Here's how the part is built. I have some questions about the finished solid (model axes, mm). Round coordinates to 2 decimals unless told otherwise and drop trailing zeros. Order: outer loops, then holes, each group sorted by start corner. A loop starts at its lowest first (then second) coordinate and runs counter-clockwise, first axis right, second up. Notation, with made-up numbers: M 32,28.25 L 46,28.25 A23 ccw 46,57.25 Z; hole C -32.5,4 d5. An arc over 180 degrees is marked long. Use one line per item in the form item = value. Start each with the question number.
```python
from build123d import *

# Parameters (mm, degrees)
CUT_EXTRUDE1_DEPTH  = 0.32
CIRPATTERN1_COUNT   = 4
DRAFT2_ANGLE        = 5
SKETCH8_R           = 0.8
BOSS_EXTRUDE1_DEPTH = 0.26
BOSS_EXTRUDE1_DRAFT = -45


with BuildPart() as part:
    # Sketch3 → Revolve1 (revolve)
    with BuildSketch(Plane(origin=(0, 0, 0), x_dir=(0, 0, -1), z_dir=(1, 0, 0)), mode=Mode.PRIVATE) as revolve1_sk:
        Polygon((-0.96, 0), (-0.96, 1.5), (-0.26, 0.8), (-0.26, 0), align=None)
    revolve(revolve1_sk.sketch.rotate(Axis((0, 0, 0.96), (0, 0, -1)), 180), axis=Axis((0, 0, 0.96), (0, 0, -1)))

    # Sketch5 → Revolve2 (revolve)
    with BuildSketch(Plane(origin=(0, 0, 0), x_dir=(0, 0, -1), z_dir=(1, 0, 0))):
        Polygon((17.04, 0), (-0.26, 0), (-0.26, 0.8), (16.7635, 0.8), (17.04, 0.5235), align=None)
    revolve(axis=Axis((0, 0, -17.04), (0, 0, 1)))

    # Sketch4 → Cut-Extrude1 (cut)
    with BuildSketch(Plane.XY.offset(0.96)):
        with BuildLine():
            Line((0, 0), (0.9271, 0))
            ThreePointArc((0.9271, 0), (0.92214099, 0.095762227), (0.907317012, 0.1905))
            Line((0.907317012, 0.1905), (0.548908506, 0.1905))
            Line((0.548908506, 0.1905), (0.295475421, 0.295475421))
            Line((0.295475421, 0.295475421), (0.1905, 0.548908506))
            Line((0.1905, 0.548908506), (0.1905, 0.907317012))
            ThreePointArc((0.1905, 0.907317012), (0.095762227, 0.92214099), (0, 0.9271))
            Line((0, 0.9271), (0, 0))
        make_face()
    cut_extrude1 = extrude(amount=-CUT_EXTRUDE1_DEPTH, mode=Mode.SUBTRACT)

    # CirPattern1: Cut-Extrude1 ×4 about axis
    cirpattern1_axis = Axis((0, 0, 0), (0, 0, 1))
    for i in range(1, CIRPATTERN1_COUNT):
        add(cut_extrude1.rotate(cirpattern1_axis, i * 360 / CIRPATTERN1_COUNT), mode=Mode.SUBTRACT)

    # Draft2
    draft2_faces = [part.faces().sort_by_distance(p)[0] for p in [
        (-0.728112759, 0.1905, 0.8),
        (-0.422191963, 0.24298771, 0.8),
        (-0.24298771, 0.422191963, 0.8),
        (-0.1905, 0.728112759, 0.8),
        (0.1905, 0.728112759, 0.8),
        (0.24298771, 0.422191963, 0.8),
        (0.422191963, 0.24298771, 0.8),
        (0.728112759, 0.1905, 0.8),
        (0.728112759, -0.1905, 0.8),
        (0.422191963, -0.24298771, 0.8),
        (0.24298771, -0.422191963, 0.8),
        (0.1905, -0.728112759, 0.8),
        (-0.1905, -0.728112759, 0.8),
        (-0.24298771, -0.422191963, 0.8),
        (-0.422191963, -0.24298771, 0.8),
        (-0.728112759, -0.1905, 0.8),
    ]]
    draft(draft2_faces, Plane(origin=(0, 0, 0.96), x_dir=(0, 1, 0), z_dir=(0, 0, 1)), DRAFT2_ANGLE)


with BuildPart() as body_2:
    # Split1: the piece on the far side of the plane
    add(part.part)
    split(bisect_by=Plane(origin=(0, 0, 0.26), x_dir=(0, -1, 0), z_dir=(0, 0, -1)), keep=Keep.BOTTOM)


with BuildPart() as part_1:
    add(part.part)

    # Split1
    split(bisect_by=Plane(origin=(0, 0, 0.26), x_dir=(0, -1, 0), z_dir=(0, 0, -1)), keep=Keep.TOP)


with BuildPart() as body_2_1:
    add(body_2.part)

    # Combine1: union part
    add(part_1.part)


with BuildPart() as boss_extrude1_tool:
    # Sketch8 → Boss-Extrude1 (with draft: the straight prism first)
    with BuildSketch(Plane.XY.offset(0.26)):
        with Locations(Location((0, 0, 0), (0, 0, 90))):
            Circle(SKETCH8_R)
    extrude(amount=-BOSS_EXTRUDE1_DEPTH)
    # Boss-Extrude1: the draft: its side faces are tilted about the plane it starts from
    boss_extrude1_sides = [boss_extrude1_tool.faces().sort_by_distance(p)[0] for p in [
        (0, -0.8, 0.13),
    ]]
    draft(boss_extrude1_sides, Plane.XY.offset(0.26), BOSS_EXTRUDE1_DRAFT)


with BuildPart() as body_2_2:
    add(body_2_1.part)

    # Boss-Extrude1: add boss_extrude1_tool
    add(boss_extrude1_tool.part)


solid = body_2_2.part
```
1) Will this pin go through, and if not, where does the flat tip stop? pin 1 Ø1 at (x, z) = (-1, -14) entering from -Y.
2) If we mould it in two halves opening along Y, with no side actions, what happens to faces 1 (the cylindrical face through (0.49, -0.63, -8.37)), 2 (the flat face through (0, 0, -17.04)), 3 (the flat face through (0, 0, 0.64))? For each: +Y half, -Y half, draft (parallel to the pull), parting line (faces both ways), or undercut.
3) If I drill on line 1 (Y direction, x = 0, z = -2.5); line 2 (Y direction, x = -0.5, z = -3.5), over which ranges is the centre line in solid material (lowest first)?
4) If we section it at A-A on z = -7: Write out the boundary of the cut face in (x, y), then the cut area to 3 significant figures.
Completed:
q1.pin_1 = -0.62
q2.face_1 = parting line
q2.face_2 = draft
q2.face_3 = undercut
q3.line_1 = -0.8 to 0.8
q3.line_2 = -0.62 to 0.62
q4.outline = C 0,0 d1.6
q4.area = 2.01 mm²
